from build123d import *

# Parameters (mm, degrees)
SKETCH027_W             = 74
SKETCH027_H             = 7
PAD018_DEPTH            = 1
SKETCH028_W             = 1
SKETCH028_H             = 7
PAD016_DEPTH            = 10
PAD016_FACE6_W          = 7
PAD016_FACE6_H          = 72
PAD019_DEPTH            = 9
SKETCH031_W             = 66
SKETCH031_H             = 7
POCKET009_DEPTH         = 9
SKETCH032_R             = 2.5
PAD020_DEPTH            = 9
SKETCH030_R             = 1.05
POCKET010_DEPTH         = 5
BODY006_PLACEMENT_ANGLE = 180


with BuildPart() as part:
    # Sketch027 → Pad018 (new body)
    with BuildSketch(Plane.XY):
        with Locations((35, 4.58)):
            Rectangle(SKETCH027_W, SKETCH027_H)
    extrude(amount=PAD018_DEPTH)

    # Sketch028 (on Face6 of Pad018) → Pad016 (join)
    with BuildSketch(Plane.XY.offset(1)):
        with Locations((-1.5, 4.58)):
            Rectangle(SKETCH028_W, SKETCH028_H)
        with Locations((71.5, 4.58)):
            Rectangle(SKETCH028_W, SKETCH028_H)
    extrude(amount=PAD016_DEPTH)

    # Pad016 Face6 → Pad019 (add)
    with BuildSketch(Plane(origin=(35, 4.58, 1), x_dir=(0, 1, 0), z_dir=(0, 0, 1))):
        Rectangle(PAD016_FACE6_W, PAD016_FACE6_H)
    extrude(amount=PAD019_DEPTH)

    # Sketch031 (on Face13 of Pad019) → Pocket009 (cut)
    with BuildSketch(Plane.XY.offset(10)):
        with Locations((35, 4.58)):
            Rectangle(SKETCH031_W, SKETCH031_H)
    extrude(amount=-POCKET009_DEPTH, mode=Mode.SUBTRACT)

    # Sketch032 (on Face7 of Pocket009) → Pad020 (join)
    with BuildSketch(Plane.XY.offset(1)):
        with Locations((34, 5.08)):
            Circle(SKETCH032_R)
    extrude(amount=PAD020_DEPTH)

    # Sketch030 (on Face26 of Pad020) → Pocket010 (cut)
    with BuildSketch(Plane.XY.offset(10)):
        with Locations((34, 5.08)):
            Circle(SKETCH030_R)
    extrude(amount=-POCKET010_DEPTH, mode=Mode.SUBTRACT)


with BuildPart() as part_1:
    # Body006 placement: moved
    add(part.part.moved(Location((75, 71, -10))).rotate(Axis((75, 71, -10), (0, 0, 1)), BODY006_PLACEMENT_ANGLE))


solid = part_1.part
Can you work these out from the model? Positions are in its coordinate system, mm. A direction names the side the tool comes from. Give positions to 0.01 mm unless a question says otherwise; leave off trailing zeros. Loops run counter-clockwise (first coordinate to the right, second up) from the corner with the lowest first, then second, coordinate; pieces in that order, holes last. Notation, with made-up numbers: M 43.5,-13 L 51.5,-13 A10 cw 51.5,-2 Z; hole C 16,59 d1. An arc over 180 degrees is marked long. One line per item, written item: value. Start each with the question number.
1) I'm going to push flat-ended pins straight in: pin 1 (1.5 mm diameter, centred on x = 5, y = 66, fed in from +Z); pin 2 (2 mm diameter, centred on x = 51.5, y = 67.5, fed in from +Z); pin 3 (5 mm diameter, centred on x = 22.5, z = -6, fed in from -Y). Where does each tip first touch, or does it pass through?
2) If we section it at B-B, the plane x = 41: Write out the boundary of the cut face in (y, z), and give its area (3 significant figures).
3) If we section it at A-A, the plane z = -4.25: Write out the boundary of the cut face in (x, y).
4) If we section it at C-C, the plane y = 65.92: Write out the boundary of the cut face in (x, z), and give its area (4 significant figures).
5) On a 3-axis mill with a long thin cutter (end or side, diameter ignored), from which of +Z, -Z, +X, -X, +Y, -Y can I reach the whole of each face in a straight line? I mean faces 4 (the face through (34.3, 62.92, -9.4)), 5 (the face through (75, 66, 0)), 6 (the face through (41, 66, -5)). Say none if no direction works.
6) Thinking about a two-plate mould opening in X: for faces 1 (the face through (6, 66, 0)), 2 (the face through (3, 66, -5)), 3 (the face through (34.3, 69.92, -9.4)), which applies, +X half, -X half, draft (parallel to the pull), parting line (faces both ways), or undercut?
7) If we section it at D-D, the plane x = 18: Write out the boundary of the cut face in (y, z), and give its area (3 significant figures).
8) If I drill on line 1 (X direction, y = 65.92, z = -1.15); line 2 (X direction, y = 64, z = -6.25); line 3 (Y direction, x = 41, z = -3.2), over which ranges is the centre line in solid material (lowest first)? Write a range as [from, to].
Completed:
1. pin 1: stops at z = 0
1. pin 2: stops at z = -9
1. pin 3: passes through
2. outline: M 62.92,-10 L 69.92,-10 L 69.92,-9 L 68.42,-9 L 68.42,0 L 66.97,0 L 66.97,-5 L 64.87,-5 L 64.87,0 L 63.42,0 L 63.42,-9 L 62.92,-9 Z
2. area: 41.5 mm^2
3. outline: M 3,62.92 L 7,62.92 L 7,69.92 L 3,69.92 Z; C 41,65.92 d5; M 73,62.92 L 77,62.92 L 77,69.92 L 73,69.92 Z; hole C 41,65.92 d2.1
4. outline: M 3,-10 L 77,-10 L 77,1 L 76,1 L 76,0 L 73,0 L 73,-9 L 43.5,-9 L 43.5,0 L 42.05,0 L 42.05,-5 L 39.95,-5 L 39.95,0 L 38.5,0 L 38.5,-9 L 7,-9 L 7,0 L 4,0 L 4,1 L 3,1 Z
4. area: 182.5 mm^2
5. face 4: +Z, -Z, +X, -X, -Y
5. face 5: +Z, +Y, -Y
5. face 6: +Z
6. face 1: undercut
6. face 2: -X half
6. face 3: draft
7. outline: M 62.92,-10 L 69.92,-10 L 69.92,-9 L 62.92,-9 Z
7. area: 7.00 mm^2
8. line 1: x = [3, 7], [38.5, 39.95], [42.05, 43.5], [73, 77]
8. line 2: x = [3, 7], [39.4, 42.6], [73, 77]
8. line 3: y = [63.42, 64.87], [66.97, 68.42]
